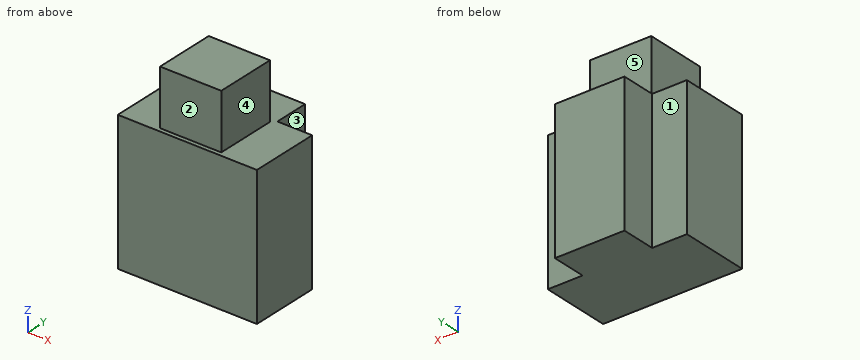
```python
from build123d import *

# Parameters (mm, degrees)
BOX_W              = 10
BOX_H              = 10
BOX_DEPTH          = 10
SKETCH_W           = 4.4
SKETCH_H           = 4.4
PAD_DEPTH          = 4
PAD_FACE4_W        = 10
PAD_FACE4_H        = 10
POCKET_DEPTH       = 2.5
POCKET_FACE5_W     = 10
POCKET_FACE5_H     = 10
POCKET001_DEPTH    = 2.5
SKETCH001_W        = 5
SKETCH001_H        = 10
PAD001_DEPTH       = 10
SKETCH002_W        = 4.4
SKETCH002_H        = 4.4
PAD002_DEPTH       = 4
PAD002_FACE22_W    = 4.4
PAD002_FACE22_H    = 4.4
POCKET002_DEPTH    = 5
POCKET002_FACE16_W = 5
POCKET002_FACE16_H = 10
POCKET003_DEPTH    = 7.5


with BuildPart() as part:
    # Box → Box (new body)
    with BuildSketch(Plane.XY):
        with Locations((5, 5)):
            Rectangle(BOX_W, BOX_H)
    extrude(amount=BOX_DEPTH)

    # Sketch (on Face6 of BaseFeature) → Pad (new body)
    with BuildSketch(Plane.XY.offset(10)):
        with Locations((5, 5)):
            Rectangle(SKETCH_W, SKETCH_H)
    extrude(amount=PAD_DEPTH)

    # Pad Face4 → Pocket (cut)
    with BuildSketch(Plane(origin=(5, 10, 5), x_dir=(1, 0, 0), z_dir=(0, 1, 0))):
        Rectangle(PAD_FACE4_W, PAD_FACE4_H)
    extrude(amount=-POCKET_DEPTH, mode=Mode.SUBTRACT)

    # Pocket Face5 → Pocket001 (cut)
    with BuildSketch(Plane(origin=(5, 0, 5), x_dir=(-1, 0, 0), z_dir=(0, -1, 0))):
        Rectangle(POCKET_FACE5_W, POCKET_FACE5_H)
    extrude(amount=-POCKET001_DEPTH, mode=Mode.SUBTRACT)

    # Sketch001 (on Face3 of Pocket001) → Pad001 (join)
    with BuildSketch(Plane(origin=(0, 7.5, 0), x_dir=(-1, 0, 0), z_dir=(0, 1, 0))):
        with Locations((-5, 5)):
            Rectangle(SKETCH001_W, SKETCH001_H)
    extrude(amount=PAD001_DEPTH)

    # Sketch002 (on Face6 of Pad001) → Pad002 (join)
    with BuildSketch(Plane.XY.offset(10)):
        with Locations((5, 12.5)):
            Rectangle(SKETCH002_W, SKETCH002_H)
    extrude(amount=PAD002_DEPTH)

    # Pad002 Face22 → Pocket002 (cut)
    with BuildSketch(Plane(origin=(5, 12.5, 14), x_dir=(0, 1, 0), z_dir=(0, 0, 1))):
        Rectangle(PAD002_FACE22_W, PAD002_FACE22_H)
    extrude(amount=-POCKET002_DEPTH, mode=Mode.SUBTRACT)

    # Pocket002 Face16 → Pocket003 (cut)
    with BuildSketch(Plane(origin=(5, 17.5, 5), x_dir=(1, 0, 0), z_dir=(0, 1, 0))):
        Rectangle(POCKET002_FACE16_W, POCKET002_FACE16_H)
    extrude(amount=-POCKET003_DEPTH, mode=Mode.SUBTRACT)


solid = part.part
```
CAD build for the part. Positions are in the model's coordinates, mm. Face numbers are marked on the shaded views. A direction names the side the tool comes from. Coordinates: 2 decimals unless noted, no trailing zeros. Order: outer loops, then holes, each group sorted by start corner. A loop starts at its lowest first (then second) coordinate and runs counter-clockwise, first axis right, second up. Notation, with made-up numbers: (12, -15.5) - (38, -15.5) arc R19 ccw to (38, 8.5) - close; hole circle Ø2 at (-14, 36). An arc over 180 degrees is marked (long way). Use a Markdown table: item, result. Add a question column.
(1) Saw through at C-C (z = 13). Give the cut face in (x, y), then the cut area to 3 significant figures.
(2) Which spindle directions (+Z, -Z, +X, -X, +Y, -Y) get a long thin tool onto all of the face, cutting with end or side? Do the marked faces 1, 2, 3, 4 and 5. Say none if no direction does.
(3) Saw through at A-A (x = 3.75). Give the cut face in (y, z), then the cut area to 3 significant figures.
(4) Saw through at D-D (x = 8.5). Give the cut face in (y, z), then the cut area to 3 significant figures.
(5) Drill centre lines: line 1 along Z through (x, y) = (9.5, 7.25); line 2 along Y through (x, z) = (9.75, 5.75); line 3 along X through (y, z) = (5.5, 10.5). Where is each one in solid material? Low to high. Write a range as [from, to].
(6) Flat gauge pins, fed straight in: pin 1 (2 mm diameter, centred on x = 2, z = 12, fed in from -Y); pin 2 (4.5 mm diameter, centred on x = 5.5, z = 13, fed in from +Y); pin 3 (3 mm diameter, centred on x = 8.5, z = 3.5, fed in from +Y); pin 4 (1.2 mm diameter, centred on y = 4, z = 12, fed in from -X). Where does each tip first touch, or does it go through?
(7) Saw through at B-B (y = 4.75). Give the cut face in (x, z).
Solved:
| question | item | result |
|---|---|---|
| 1 | outline | (2.8, 2.8) - (7.2, 2.8) - (7.2, 7.2) - (2.8, 7.2) - close |
| 1 | area | 19.4 mm² |
| 2 | face 1 | +Z, -Z, -X, +Y |
| 2 | face 2 | +Z, +X, -X, -Y |
| 2 | face 3 | +Z, -Z, +X, +Y |
| 2 | face 4 | +Z, +X, +Y, -Y |
| 2 | face 5 | +Z, +X, -X, +Y |
| 3 | outline | (2.5, 0) - (10, 0) - (10, 10) - (7.2, 10) - (7.2, 14) - (2.8, 14) - (2.8, 10) - (2.5, 10) - close |
| 3 | area | 92.6 mm² |
| 4 | outline | (2.5, 0) - (7.5, 0) - (7.5, 10) - (2.5, 10) - close |
| 4 | area | 50.0 mm² |
| 5 | line 1 | z = [0, 10] |
| 5 | line 2 | y = [2.5, 7.5] |
| 5 | line 3 | x = [2.8, 7.2] |
| 6 | pin 1 | stops at y = 2.8 |
| 6 | pin 2 | stops at y = 7.2 |
| 6 | pin 3 | stops at y = 10 |
| 6 | pin 4 | stops at x = 2.8 |
| 7 | outline | (0, 0) - (10, 0) - (10, 10) - (7.2, 10) - (7.2, 14) - (2.8, 14) - (2.8, 10) - (0, 10) - close |
